Could you check a few things on this model? Use its own coordinates, in mm. Face numbers are marked on the shaded views. A direction names the side the tool comes from. Give positions to 0.01 mm unless a question says otherwise; leave off trailing zeros. Loops run counter-clockwise (first coordinate to the right, second up) from the corner with the lowest first, then second, coordinate; pieces in that order, holes last. Notation, with made-up numbers: (61.5, 49.25) - (69.5, 49.25) arc R22 ccw to (69.5, 62.25) - close; hole circle Ø4 at (35.5, 44). An arc over 180 degrees is marked (long way). Use CSV: the item, a comma, the result in double quotes.
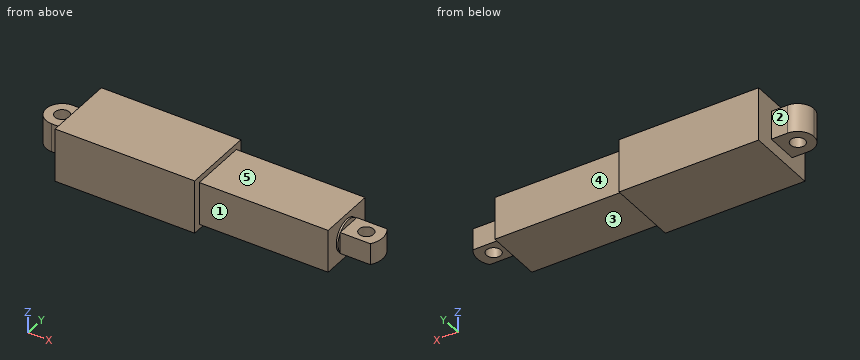
from build123d import *

# Parameters (mm, degrees)
SKETCH_1_W           = 39
SKETCH_1_H           = 20
EXTRUDE_1_DEPTH      = 15
SKETCH_2_W           = 8
SKETCH_2_H           = 9
EXTRUDE_2_DEPTH      = 9
SKETCH_3_R           = 2.025
CUT_EXTRUDE_1_DEPTH  = 10
FILLET_1_R           = 4.5
SKETCH_4_W           = 12
SKETCH_4_H           = 16
EXTRUDE_3_DEPTH      = 36
SKETCH_5_R           = 4.5
EXTRUDE_4_DEPTH      = 0.5
EXTRUDE_5_DEPTH      = 3
EXTRUDE_5_DEPTH_BACK = 3
SKETCH_7_R           = 2.025


with BuildPart() as part:
    # 스케치1 → 보스-돌출1 (new body)
    with BuildSketch(Plane.XY):
        Rectangle(SKETCH_1_W, SKETCH_1_H)
    extrude(amount=EXTRUDE_1_DEPTH)

    # 스케치2 → 보스-돌출2 (add)
    with BuildSketch(Plane.ZY.offset(19.5)):
        with Locations((7.5, 0)):
            Rectangle(SKETCH_2_W, SKETCH_2_H)
    extrude(amount=EXTRUDE_2_DEPTH)

    # 스케치3 → 컷-돌출1 (cut)
    with BuildSketch(Plane.XY.offset(11.5)):
        with Locations((-24, 0)):
            Circle(SKETCH_3_R)
    extrude(amount=-CUT_EXTRUDE_1_DEPTH, mode=Mode.SUBTRACT)

    # 필렛1
    fillet_1_edges = [part.edges().sort_by_distance(p)[0] for p in [
        (-28.5, -4.5, 7.5),
        (-28.5, 4.5, 7.5),
    ]]
    fillet(fillet_1_edges, radius=FILLET_1_R - 0.0001)  # a hair under: the kernel refuses the full size

    # 스케치4 → 보스-돌출3 (add)
    with BuildSketch(Plane(origin=(19.5, 0, 0), x_dir=(0, 0, -1), z_dir=(1, 0, 0))):
        with Locations((-7.366003783, 0)):
            Rectangle(SKETCH_4_W, SKETCH_4_H)
    extrude(amount=EXTRUDE_3_DEPTH)

    # 스케치5 → 보스-돌출4 (add)
    with BuildSketch(Plane(origin=(55.5, 0, 0), x_dir=(0, 0, -1), z_dir=(1, 0, 0))):
        with Locations((-7.366003783, 0)):
            Circle(SKETCH_5_R)
    extrude(amount=EXTRUDE_4_DEPTH)

    # 스케치7 → 보스-돌출5 (add, two sides: drawn at the far end of the back side and taken through both)
    with BuildSketch(Plane.XY.offset(7.366003783).offset(-EXTRUDE_5_DEPTH_BACK)):
        with BuildLine():
            Line((56, -3.604783634), (64.44555705, -3.604783634))
            ThreePointArc((64.44555705, -3.604783634), (65.594419255, 0), (64.44555705, 3.604783634))
            Line((64.44555705, 3.604783634), (56, 3.604783634))
            Line((56, 3.604783634), (56, -3.604783634))
        make_face()
        with Locations((61, 0)):
            Circle(SKETCH_7_R, mode=Mode.SUBTRACT)
    extrude(amount=EXTRUDE_5_DEPTH + EXTRUDE_5_DEPTH_BACK)


solid = part.part
1) Suppose I cut it at A-A (x = 61). Please give me the cut outline in (y, z) (3 decimals).
Answer below:
outline,"(-3.605, 4.366) - (-2.025, 4.366) - (-2.025, 10.366) - (-3.605, 10.366) - close; (2.025, 4.366) - (3.605, 4.366) - (3.605, 10.366) - (2.025, 10.366) - close"
2) I need wall thicknesses on line 1 along Y through (x, z) = (61, 8.8) (3 decimals); line 2 along Y through (x, z) = (-24, 7) (3 decimals); line 3 along Z through (x, y) = (26, -1.25). Which ranges of each line are inside material? Lowest first, please.
Answer below:
line 1,"y = -3.605 to -2.025, 2.025 to 3.605"
line 2,"y = -4.5 to -2.025, 2.025 to 4.5"
line 3,"z = 1.37 to 13.37"
3) Suppose I cut it at B-B (z = 8.5). State how many separate pieces and enclosed holes the cut face has, plus the area to 3 significant figures.
Answer below:
separate pieces,"1"
enclosed holes,"2"
area,"1,470 mm2"
4) Which directions (+Z, -Z, +X, -X, +Y, -Y) give clear straight access to the entire face, cutting with the end or side of a thin tool? Please do the marked faces 1, 2, 3, 4 and 5.
Answer below:
face 1,"+Z, -Z, +X, -Y"
face 2,"+Z, -Z, -X, +Y"
face 3,"-Z, +X, +Y, -Y"
face 4,"+Z, -Z, +X, +Y"
face 5,"+Z, +X, +Y, -Y"
5) I'm going to push flat-ended pins straight in: P1, Ø8, axis at x = 61.5, y = 0, coming from the +Z side; P2, Ø8, axis at x = 32.5, z = 6, coming from the -Y side; P3, Ø1.2, axis at y = -1, z = 3.5, coming from the +X side. Where does each tip first touch, or does it pass through?
Answer below:
P1,"stops at z = 10.37"
P2,"stops at y = -8"
P3,"stops at x = 56"
